Could you check a few things on this model? Use its own coordinates, in mm. Give positions to 0.01 mm unless a question says otherwise; leave off trailing zeros. Order: outer loops, then holes, each group sorted by start corner. A loop starts at its lowest first (then second) coordinate and runs counter-clockwise, first axis right, second up. Notation, with made-up numbers: (50, 56) -> (65, 56) arc R13 ccw to (65, 79) -> close; hole circle Ø2 at (-14, -26.5). An arc over 180 degrees is marked (long way). Use one line per item in the form item = value. Start each with the question number.
Autodesk Inventor part; units mm, degrees
ref_plane "YZ Plane" through (0, 0, 0) normal (1, 0, 0) x (0, 1, 0)
ref_plane "XZ Plane" through (0, 0, 0) normal (0, 1, 0) x (-1, 0, 0)
ref_plane "XY Plane" through (0, 0, 0) normal (0, 0, 1) x (1, 0, 0)
sketch "Szkic1" plane through (0, 0, 0) normal (0, 0, 1) x (1, 0, 0)
  line L0 (-30, 58) -> (30, 58)
  circle A0 centre (0, 0) radius 15
  line L1 (0, 0) -> (30, 0)
  line L2 (30, 0) -> (30, 58)
  line L3 (-30, 0) -> (-30, 58)
  line L4 (-30, 0) -> (-30, -20)
  line L5 (-30, -20) -> (30, -20)
  line L6 (30, -20) -> (30, 0)
  dimension "d2" = 30
  dimension "d7" = 78
  dimension "d8" = 60
  dimension "d9" = 20
extrude "Wyciągnięcie proste1" add sketch "Szkic1" along normal blind 8
sketch "Szkic2" plane through (0, 0, 8) normal (0, 0, 1) x (1, 0, 0)
  line L0 (30, 58) -> (-30, 58)
  line L1 (-30, 58) -> (-30, 18)
  line L2 (-30, 58) -> (-30, -20)
  line L3 (-30, 18) -> (30, 18)
  line L4 (30, -20) -> (30, 58)
  line L5 (30, 18) -> (30, 58)
  line L6 (-30, 58) -> (-30, 48)
  line L7 (-30, 18) -> (-30, 28)
  line L8 (-30, 28) -> (30, 28)
  line L9 (-30, 48) -> (30, 48)
  line L10 (-30, 48) -> (-15, 48)
  line L11 (-15, 48) -> (-15, 28)
  line L12 (30, 48) -> (15, 48)
  line L13 (15, 48) -> (15, 28)
  circle A0 centre (-15, 48) radius 2.5
  circle A1 centre (15, 48) radius 2.5
  circle A2 centre (-15, 28) radius 2.5
  circle A3 centre (15, 28) radius 2.5
  point P0 (0, 0)
  dimension "d12" = 40
  dimension "d13" = 90
  dimension "d14" = 10
  dimension "d15" = 10
  dimension "d16" = 15
  dimension "d17" = 15
  dimension "d18" = 5
  dimension "d19" = 5
  dimension "d20" = 5
  dimension "d21" = 5
extrude "Wyciągnięcie proste2" cut sketch "Szkic2" against normal up to next contours A1 L13 L9 | L9 A1 | A0 L9 | L9 L11 A0 | A3 L8 | L8 L13 A3 | L13 A1 L9 | A2 L11 L8 | L8 A2 | L9 A0 L11 | L8 A3 L13 | L11 A2 L8
sketch "Szkic3" plane through (0, 0, 0) normal (0, 0, -1) x (-1, 0, 0)
  circle A0 centre (0, 0) radius 15
  line L0 (-30, -20) -> (30, -20)
  line L1 (30, -20) -> (30, 18)
  line L2 (30, 18) -> (-30, 18)
  line L3 (-30, 18) -> (-30, -20)
  line L4 (-30, 18) -> (-30, -20)
  line L5 (-30, 18) -> (-22, 18)
  line L6 (30, 18) -> (-30, 18)
  line L7 (-22, 18) -> (-22, -20)
  line L8 (30, 18) -> (22, 18)
  line L9 (22, 18) -> (22, -20)
  line L10 (-22, 18) -> (-22, 10)
  line L11 (-22, -20) -> (-22, -12)
  line L12 (22, 18) -> (22, 10)
  line L13 (22, -20) -> (22, -12)
  circle A1 centre (-22, 10) radius 2.5
  circle A2 centre (-22, -12) radius 2.5
  circle A3 centre (22, 10) radius 2.5
  circle A4 centre (22, -12) radius 2.5
  circle A5 centre (-15, 28) radius 2.5
  circle A6 centre (-15, 48) radius 2.5
  circle A7 centre (15, 48) radius 2.5
  circle A8 centre (15, 28) radius 2.5
  circle A9 centre (0, 0) radius 15
  line L14 (30, 58) -> (-30, 58)
  line L15 (-30, 58) -> (-30, -20)
  line L16 (-30, -20) -> (30, -20)
  line L17 (30, -20) -> (30, 58)
  point P0 (0, -1)
  dimension "d24" = 8
  dimension "d25" = 8
  dimension "d26" = 8
  dimension "d27" = 8
  dimension "d28" = 8
  dimension "d29" = 8
  dimension "d30" = 5
  dimension "d31" = 5
  dimension "d32" = 5
  dimension "d33" = 5
extrude "Wyciągnięcie proste3" cut sketch "Szkic3" against normal up to next contours A2 L7 | L7 A2 | A4 L9 | L9 A4 | A1 L7 | L7 A1 | A3 L9 | L9 A3
thread "Gwint1"
thread "Gwint2"
thread "Gwint3"
thread "Gwint4"
properties part number "Uchwyt silnika krokowego osi Y - płaski"
(1) We'd pull the mould along Y, two halves only. Please class faces 1 (the cylindrical face through (24, -13.5, 3.9)), 2 (the flat face through (0, -20, 4)), 3 (the flat face through (-30, 18, 4)): pulls with the +Y half, pulls with the -Y half, needs draft (parallel to the pull), parting line crosses it, or undercut.
(2) I'm going to push a flat-ended pin straight in: pin 1 Ø3 at (x, y) = (15, 48) entering from -Z. Where does the tip first touch, or does it pass through?
(3) Please list where these lines run through material, in increasing order: probe 1 along Y at (x, z) = (22, 2.5); probe 2 along X at (y, z) = (26, 1.5); probe 3 along X at (y, z) = (9, 2.75).
(4) Imagine slicing it at A-A (y = 48). Write out the boundary of the cut face in (x, z).
(5) Imagine slicing it at D-D (y = -12). Write out the boundary of the cut face in (x, z), plus the area to 3 significant figures.
(6) Imagine slicing it at B-B (x = 22). Write out the boundary of the cut face in (y, z), plus the area to 3 significant figures.
(7) Imagine slicing it at C-C (z = 1.25). Give the number of separate pieces and of enclosed holes in the cut face, plus the area to 3 significant figures.
Calculated:
q1.face_1 = undercut
q1.face_2 = pulls with the -Y half
q1.face_3 = needs draft
q2.pin_1 = through
q3.probe_1 = -20 to -14.5, -9.5 to 7.5, 12.5 to 58
q3.probe_2 = -30 to -16.5, -13.5 to 13.5, 16.5 to 30
q3.probe_3 = -30 to -24.29, -19.71 to -12, 12 to 19.71, 24.29 to 30
q4.outline = (-30, 0) -> (-17.5, 0) -> (-17.5, 8) -> (-30, 8) -> close; (-12.5, 0) -> (12.5, 0) -> (12.5, 8) -> (-12.5, 8) -> close; (17.5, 0) -> (30, 0) -> (30, 8) -> (17.5, 8) -> close
q5.outline = (-30, 0) -> (-24.5, 0) -> (-24.5, 8) -> (-30, 8) -> close; (-19.5, 0) -> (-9, 0) -> (-9, 8) -> (-19.5, 8) -> close; (9, 0) -> (19.5, 0) -> (19.5, 8) -> (9, 8) -> close; (24.5, 0) -> (30, 0) -> (30, 8) -> (24.5, 8) -> close
q5.area = 256 mm2
q6.outline = (-20, 0) -> (-14.5, 0) -> (-14.5, 8) -> (-20, 8) -> close; (-9.5, 0) -> (7.5, 0) -> (7.5, 8) -> (-9.5, 8) -> close; (12.5, 0) -> (58, 0) -> (58, 8) -> (12.5, 8) -> close
q6.area = 544 mm2
q7.separate_pieces = 1
q7.enclosed_holes = 9
q7.area = 3,820 mm2
